Can you work these out from the model? Positions are in its coordinate system, mm. Coordinates: 2 decimals unless noted, no trailing zeros. Order: outer loops, then holes, each group sorted by start corner. A loop starts at its lowest first (then second) coordinate and runs counter-clockwise, first axis right, second up. Notation, with made-up numbers: (12, 73.5) - (32, 73.5) arc R29 cw to (32, 94.5) - close; hole circle Ø3 at (29, 46.5). An arc over 180 degrees is marked (long way). Use a Markdown table: item, result. Add a question column.
(1) We'd pull the mould along X, two halves only. Please class faces 1 (the cylindrical face through (-190.763, -3.83, -0.07)), 2 (the cylindrical face through (212.15, -11.99, 0.07)), 3 (the flat face through (3, 0, -5)), 4 (the flat face through (-215, 0, 0)): pulls with the +X half, pulls with the -X half, needs draft (parallel to the pull), parting line crosses it, or undercut.
(2) If I drill on L1, parallel to X at y = -0.5, z = -1; L2, parallel to X at y = 8.5, z = -3.75; L3, parallel to Y at x = 200, z = -1.75, over which ranges is the centre line in solid material (lowest first)? Write a range as [from, to].
(3) I want a section at B-B (y = 0). List the corners of the cut face in (x, z) for me.
(4) I want a section at C-C (z = -0.5). List the corners of the cut face in (x, y) for me, and give its area (3 significant figures).
(5) I want a section at A-A (x = -200). List the corners of the cut face in (y, z) for me, and give its area (3 significant figures).
```python
from build123d import *

# Parameters (mm, degrees)
CROQUIS1_R              = 10
SALIENTE_EXTRUIR2_DEPTH = 5


with BuildPart() as part:
    # Croquis1 → Saliente-Extruir2 (new body, symmetric)
    with BuildSketch(Plane.XY):
        with BuildLine():
            Line((-205, 15), (205, 15))
            ThreePointArc((205, 15), (212.071067812, 12.071067812), (215, 5))
            Line((215, 5), (215, -5))
            ThreePointArc((215, -5), (212.071067812, -12.071067812), (205, -15))
            Line((205, -15), (-205, -15))
            ThreePointArc((-205, -15), (-212.071067812, -12.071067812), (-215, -5))
            Line((-215, -5), (-215, 5))
            ThreePointArc((-215, 5), (-212.071067812, 12.071067812), (-205, 15))
        make_face()
        with Locations((-200, 0)):
            Circle(CROQUIS1_R, mode=Mode.SUBTRACT)
        with Locations((200, 0)):
            Circle(CROQUIS1_R, mode=Mode.SUBTRACT)
    extrude(amount=SALIENTE_EXTRUIR2_DEPTH, both=True)


solid = part.part
```
Answers follow:
| question | item | result |
|---|---|---|
| 1 | face 1 | undercut |
| 1 | face 2 | pulls with the +X half |
| 1 | face 3 | needs draft |
| 1 | face 4 | pulls with the -X half |
| 2 | L1 | x = [-215, -209.99], [-190.01, 190.01], [209.99, 215] |
| 2 | L2 | x = [-214.37, -205.27], [-194.73, 194.73], [205.27, 214.37] |
| 2 | L3 | y = [-15, -10], [10, 15] |
| 3 | outline | (-215, -5) - (-210, -5) - (-210, 5) - (-215, 5) - close; (-190, -5) - (190, -5) - (190, 5) - (-190, 5) - close; (210, -5) - (215, -5) - (215, 5) - (210, 5) - close |
| 4 | outline | (-215, -5) arc R10 ccw to (-205, -15) - (205, -15) arc R10 ccw to (215, -5) - (215, 5) arc R10 ccw to (205, 15) - (-205, 15) arc R10 ccw to (-215, 5) - close; hole circle Ø20 at (-200, 0); hole circle Ø20 at (200, 0) |
| 4 | area | 12,200 mm² |
| 5 | outline | (-15, -5) - (-10, -5) - (-10, 5) - (-15, 5) - close; (10, -5) - (15, -5) - (15, 5) - (10, 5) - close |
| 5 | area | 100 mm² |
